from build123d import *

# Parameters (mm, degrees)
F0_W     = 203.2
F0_H     = 38.1
F1_DEPTH = 19.05
F2_R     = 19.04999
F4_DEPTH = 12.7
F5_R     = 4.7625
F6_DEPTH = 12.7


# Not quite as in the source:
# - a fillet or chamfer is up to 0.001 mm smaller than in the source, because OpenCascade refuses the exact size


with BuildPart() as f1:
    # F0 (on Front) → F1 (new body, symmetric)
    with BuildSketch(Plane.XZ):
        Rectangle(F0_W, F0_H)
    extrude(amount=F1_DEPTH, both=True)

    # F2 (radius 19.05 in the source; OpenCascade refuses exactly that, so slightly less here)
    f2_edges = [f1.edges().sort_by_distance(p)[0] for p in [
        (0, -19.05, 19.05),
        (0, 19.05, 19.05),
        (0, 19.05, -19.05),
        (0, -19.05, -19.05),
    ]]
    fillet(f2_edges, radius=F2_R)

    # F3 (on Front) → F4 (join, symmetric)
    with BuildSketch(Plane.XZ):
        with BuildLine():
            Line((-101.6, -19.0500002354), (-101.6, 0))
            Line((-101.6, 0), (-101.6, 19.05))
            ThreePointArc((-101.6, 19.05), (-120.9801457995, -1.177e-07), (-101.6, -19.0500002354))
        make_face()
        with BuildLine():
            Line((101.6, 19.05), (101.6, 0))
            Line((101.6, 0), (101.6, -19.0500002354))
            ThreePointArc((101.6, -19.0500002354), (121.1996012404, -1.177e-07), (101.6, 19.05))
        make_face()
    extrude(amount=F4_DEPTH, both=True)

    # F5 (on Front) → F6 (cut, symmetric)
    with BuildSketch(Plane.XZ):
        with Locations((-107.95, 0)):
            Circle(F5_R)
        with BuildLine():
            ThreePointArc((112.7125, 0), (107.95, 4.7625), (103.1875, 0))
            ThreePointArc((103.1875, 0), (107.95, -4.7625), (112.7125, 0))
        make_face()
    extrude(amount=F6_DEPTH, both=True, mode=Mode.SUBTRACT)


solid = f1.part
Build history of the part. All positions in model axes, mm. A direction names the side the tool comes from. Round coordinates to 2 decimals unless told otherwise and drop trailing zeros. Loops run counter-clockwise (first coordinate to the right, second up) from the corner with the lowest first, then second, coordinate; pieces in that order, holes last. Notation, with made-up numbers: (-18.75, 63) -> (5.25, 63) arc R22 cw to (5.25, 97) -> close; hole circle Ø9 at (19.5, -0.5). An arc over 180 degrees is marked (long way). One line per item, written item: value. Start each with the question number.
Q1. Cut at A-A on x = -107.95. List the corners of the cut face in (y, z).
Q2. Cut at B-B on y = 3. Count the separate pieces of the cut face and the enclosed holes in it, plus the area to 3 significant figures.
Q3. Probe line 1 along X through (y, z) = (8, 3); line 2 along Z through (x, y) = (-107, 8); line 3 along Y through (x, z) = (109, 14.5). List the from-to ranges inside material, lowest first.
Q4. Two-plate mould, pull along X, no slides. Class faces 1 (the face through (101.6, 15, 0)), 2 (the face through (113, -12.7, 0)), 3 (the face through (101.6, 10, 18)), 4 (the face through (1.42, -13.62, -13.32)): released by +X, released by -X, zero draft, split by the parting line, or undercut.
Q5. Drop flat-ended pins along their axis: pin 1 Ø12 at (x, y) = (-39, 0.5) entering from +Z; pin 2 Ø6 at (y, z) = (14, 0) entering from +X; pin 3 Ø11 at (x, z) = (107.95, 0) entering from +Y. Give the stop position or say it passes through.
Q6. Cut at C-C on z = -2.5. List the corners of the cut face in (x, y), plus the area to 3 significant figures.
Q7. 3-axis set-ups, long thin cutter, end or side, ignore diameter. For faces 5 (the face through (-101.6, -15, 0)), 6 (the face through (-101.6, 15, 0)), 7 (the face through (-101.6, -10, -18)), 8 (the face through (101.6, -10, 18)): which of +Z, -Z, +X, -X, +Y, -Y reach the whole face in a straight line?
Computed:
1. outline: (-12.7, -18.08) -> (12.7, -18.08) -> (12.7, -4.76) -> (-12.7, -4.76) -> close; (-12.7, 4.76) -> (12.7, 4.76) -> (12.7, 18.08) -> (-12.7, 18.08) -> close
2. separate pieces: 1
2. enclosed holes: 2
2. area: 8,680 mm²
3. line 1: -120.74 to -111.65, -104.25 to 104.25, 111.65 to 120.96
3. line 2: -18.37 to -4.67, 4.67 to 18.37
3. line 3: -12.7 to 12.7
4. face 1: released by +X
4. face 2: zero draft
4. face 3: undercut
4. face 4: undercut
5. pin 1: z = 19.05
5. pin 2: x = 121.2
5. pin 3: y = 12.7
6. outline: (-120.82, -12.7) -> (-112, -12.7) -> (-112, 12.7) -> (-120.82, 12.7) -> close; (-103.9, -12.7) -> (-101.6, -12.7) -> (-101.6, -18.89) -> (101.6, -18.89) -> (101.6, -12.7) -> (103.9, -12.7) -> (103.9, 12.7) -> (101.6, 12.7) -> (101.6, 18.89) -> (-101.6, 18.89) -> (-101.6, 12.7) -> (-103.9, 12.7) -> close; (112, -12.7) -> (121.03, -12.7) -> (121.03, 12.7) -> (112, 12.7) -> close
6. area: 8,240 mm²
7. face 5: +Z, -Z, -X, -Y
7. face 6: +Z, -Z, -X, +Y
7. face 7: -Z, -Y
7. face 8: +Z, -Y
